Source: CAD feature listing. Evaluate the final solid. Frame: model axes, mm. A direction names the side the tool comes from. Round coordinates to 2 decimals unless told otherwise and drop trailing zeros. Order: outer loops, then holes, each group sorted by start corner. A loop starts at its lowest first (then second) coordinate and runs counter-clockwise, first axis right, second up. Notation, with made-up numbers: (24, 37) - (66, 37) arc R8 cw to (66, 42) - close; hole circle Ø8 at (37.25, 61.25). An arc over 180 degrees is marked (long way). Return JSON: item names as keys, results as strings. Group by question number.
1) Section C-C, the plane x = 12.5. Return loops of the section in (y, z), plus the area to 3 significant figures.
2) Access query for faces 5 (the flat face through (0, 17, 0)), 6 (the cylindrical face through (10.699, -5.715, 0.017)), 7 (the flat face through (14, 1, 0)). Directions: +Z, -Z, +X, -X, +Y, -Y. A direction counts if a zero-diameter tool reaches every point of the face in a straight line with its end or side. Return the directions, or none.
3) Mould query, pull axis Y, two halves, no side actions, for faces 1 (the flat face through (-7, -1, 0)), 2 (the cylindrical face through (14.15, -13.99, 0.02)), 3 (the flat face through (0, 11, 0)), 4 (the cylindrical face through (12, -2.4, -1.9)). Classes: pulls with the +Y half, pulls with the -Y half, needs draft (parallel to the pull), parting line crosses it, or undercut.
4) Section B-B, the plane x = -1.5. Return loops of the section in (y, z), plus the area to 3 significant figures.
5) Section D-D, the plane z = -2.05. Return loops of the section in (x, y).
6) Contact query for flat-ended pins moving along their axis: P1, Ø1.2, axis at x = -7.5, z = 0, coming from the +Y side; P2, Ø2, axis at x = 8.5, y = 6.5, coming from the -Z side; P3, Ø2, axis at x = 4, z = -3.5, coming from the +Y side; P4, Ø3.5, axis at x = 9, y = -3, coming from the -Z side. Output: stop coordinate, or through.
7) Section A-A, the plane y = 1.5. Return loops of the section in (x, z).
8) Ray query, line 1 (X direction, y = 2.5, z = 0.95); line 2 (Y direction, x = -1.5, z = 0.7); line 3 (Y direction, x = 9.5, z = 0.5). Return the intervals inside material, ascending. Write a range as from..to.
```python
from build123d import *

# Parameters (mm, degrees)
BOSS_EXTRUDE2_DEPTH     = 1.2
BOSS_EXTRUDE3_DEPTH     = 5
CUT_EXTRUDE1_DEPTH      = 25.828209762
CUT_EXTRUDE1_DEPTH_BACK = 25.828209762


with BuildPart() as part:
    # Sketch1 → Boss-Extrude2 (new, symmetric)
    with BuildSketch(Plane.XY):
        with BuildLine():
            ThreePointArc((7, 17), (14.071067812, 14.071067812), (17, 7))
            Line((17, 7), (17, -7))
            ThreePointArc((17, -7), (14.071067812, -14.071067812), (7, -17))
            Line((7, -17), (-7, -17))
            ThreePointArc((-7, -17), (-14.071067812, -14.071067812), (-17, -7))
            Line((-17, -7), (-17, 7))
            ThreePointArc((-17, 7), (-14.071067812, 14.071067812), (-7, 17))
            Line((-7, 17), (7, 17))
        make_face()
        with BuildLine():
            Line((-7, 14), (7, 14))
            ThreePointArc((7, 14), (11.949747468, 11.949747468), (14, 7))
            Line((14, 7), (14, -4.4))
            ThreePointArc((14, -4.4), (12.535533906, -7.935533906), (9, -9.4))
            Line((9, -9.4), (6, -9.4))
            ThreePointArc((6, -9.4), (4.585786438, -8.814213562), (4, -7.4))
            Line((4, -7.4), (4, 2.4))
            ThreePointArc((4, 2.4), (4.292893219, 3.107106781), (5, 3.4))
            Line((5, 3.4), (6, 3.4))
            ThreePointArc((6, 3.4), (6.707106781, 3.107106781), (7, 2.4))
            Line((7, 2.4), (7, -5))
            ThreePointArc((7, -5), (7.292893219, -5.707106781), (8, -6))
            Line((8, -6), (10, -6))
            ThreePointArc((10, -6), (10.707106781, -5.707106781), (11, -5))
            Line((11, -5), (11, 7))
            ThreePointArc((11, 7), (9.828427125, 9.828427125), (7, 11))
            Line((7, 11), (-7, 11))
            ThreePointArc((-7, 11), (-9.828427125, 9.828427125), (-11, 7))
            Line((-11, 7), (-11, -5))
            ThreePointArc((-11, -5), (-10.707106781, -5.707106781), (-10, -6))
            Line((-10, -6), (-8, -6))
            ThreePointArc((-8, -6), (-7.292893219, -5.707106781), (-7, -5))
            Line((-7, -5), (-7, 2.4))
            ThreePointArc((-7, 2.4), (-6.707106781, 3.107106781), (-6, 3.4))
            Line((-6, 3.4), (-5, 3.4))
            ThreePointArc((-5, 3.4), (-4.292893219, 3.107106781), (-4, 2.4))
            Line((-4, 2.4), (-4, -7.4))
            ThreePointArc((-4, -7.4), (-4.585786438, -8.814213562), (-6, -9.4))
            Line((-6, -9.4), (-9, -9.4))
            ThreePointArc((-9, -9.4), (-12.535533906, -7.935533906), (-14, -4.4))
            Line((-14, -4.4), (-14, 7))
            ThreePointArc((-14, 7), (-11.949747468, 11.949747468), (-7, 14))
        make_face(mode=Mode.SUBTRACT)
    extrude(amount=BOSS_EXTRUDE2_DEPTH, both=True)

    # Sketch2 → Boss-Extrude3 (add)
    with BuildSketch(Plane(origin=(0, 0, -1.2), x_dir=(-1, 0, 0), z_dir=(0, 0, -1))):
        with BuildLine():
            Line((-10.570714214, -6), (10.570714214, -6))
            ThreePointArc((10.570714214, -6), (12, -2.5), (10.570714214, 1))
            Line((10.570714214, 1), (-10.570714214, 1))
            ThreePointArc((-10.570714214, 1), (-12, -2.5), (-10.570714214, -6))
        make_face()
    extrude(amount=BOSS_EXTRUDE3_DEPTH)

    # Sketch3 → Cut-Extrude1 (cut, two sides: drawn at the far end of the back side and taken through both)
    with BuildSketch(Plane(origin=(0, 0, 0), x_dir=(1, 0, 0), z_dir=(0, 1, 0)).offset(-CUT_EXTRUDE1_DEPTH_BACK)):
        Polygon((-4.901923789, 4.2), (-7.5, 2.7), (-12, 2.7), (-15.905472788, 2.7), (-15.905472788, 4.2), (-15.905472788, 10.094032112), (14.61063782, 10.094032112), (14.61063782, 4.2), (14.61063782, 2.7), (12, 2.7), (7.5, 2.7), (4.901923789, 4.2), align=None)
        Polygon((4.901923789, 2.7), (-4.901923789, 2.7), (-7.5, 1.2), (7.5, 1.2), align=None)
    extrude(amount=CUT_EXTRUDE1_DEPTH + CUT_EXTRUDE1_DEPTH_BACK, mode=Mode.SUBTRACT)


solid = part.part
```
Geometry check:
{
 "1": {"outline": "(-15.35, -1.2) - (-7.97, -1.2) - (-7.97, 1.2) - (-15.35, 1.2) - close; (11.33, -1.2) - (15.35, -1.2) - (15.35, 1.2) - (11.33, 1.2) - close", "area": "27.4 mm2"},
 "2": {"face 5": "+Z, -Z, +X, -X, +Y", "face 6": "+Z", "face 7": "+Z, -Z"},
 "3": {"face 1": "undercut", "face 2": "pulls with the -Y half", "face 3": "undercut", "face 4": "parting line crosses it"},
 "4": {"outline": "(-17, -1.2) - (11, -1.2) - (11, 1.2) - (-17, 1.2) - close; (-6, -4.2) - (1, -4.2) - (1, -2.7) - (-6, -2.7) - close; (14, -1.2) - (17, -1.2) - (17, 1.2) - (14, 1.2) - close", "area": "84.9 mm2"},
 "5": {"outline": "(-10.57, -6) - (-6.03, -6) - (-6.03, 1) - (-10.57, 1) arc R5 ccw to start; (6.03, -6) - (10.57, -6) arc R5 ccw to (10.57, 1) - (6.03, 1) - close"},
 "6": {"P1": "y = 17", "P2": "z = -1.2", "P3": "y = 1", "P4": "z = -2.84"},
 "7": {"outline": "(-17, -1.2) - (-14, -1.2) - (-14, 1.2) - (-17, 1.2) - close; (-11, -1.2) - (-7, -1.2) - (-7, 1.2) - (-11, 1.2) - close; (-4, -1.2) - (4, -1.2) - (4, 1.2) - (-4, 1.2) - close; (7, -1.2) - (11, -1.2) - (11, 1.2) - (7, 1.2) - close; (14, -1.2) - (17, -1.2) - (17, 1.2) - (14, 1.2) - close"},
 "8": {"line 1": "-17..-14, -11..-6.99, -4.01..4.01, 6.99..11, 14..17", "line 2": "-17..11, 14..17", "line 3": "-16.68..-9.37, -6..10.12, 13.54..16.68"}
}
